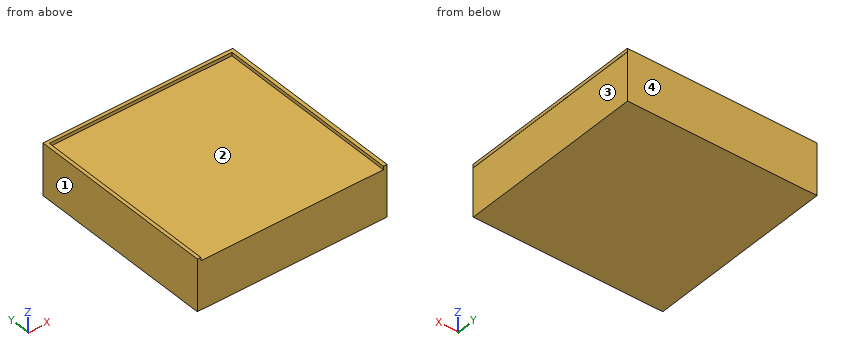
```python
from build123d import *

# Parameters (mm, degrees)
F2_DEPTH = 1
F0_W     = 55
F0_H     = 55
F3_DEPTH = 14


with BuildPart() as f2:
    # F1 (on face) → F2 (new body)
    with BuildSketch(Plane.XY):
        Polygon((1, -1), (54, -1), (54, -55), (55.060755, -55), (55.060755, 0), (0, 0), (0, -55), (1, -55), align=None)
    extrude(amount=F2_DEPTH)

    # F0 (on Top) → F3 (join)
    with BuildSketch(Plane.XY):
        with Locations((27.5, -27.5)):
            Rectangle(F0_W, F0_H)
    extrude(amount=-F3_DEPTH)


solid = f2.part
```
Geometry check sheet. Reference: the model listing, model coordinates, mm. Face numbers are marked on the shaded views. Coordinates: 2 decimals unless noted, no trailing zeros. Write each loop counter-clockwise with the first axis right and the second up, starting at its lowest first coordinate (ties: lowest second). Pieces come first, ordered by that corner, then holes. Notation, with made-up numbers: (81.5, 71) -> (99.5, 71) arc R34 ccw to (99.5, 108) -> close; hole circle Ø6 at (82.25, 30). An arc over 180 degrees is marked (long way). Use CSV: the item, a comma, the result in double quotes. Start each with the question number.
Item 1: Cross-section at B-B, the plane x = 12. Record the cut outline in (y, z).
Item 2: Thickness scan on line 1 (X direction, y = -35.5, z = -10.25); line 2 (Z direction, x = 2, y = -22). Record the ranges inside material, lowest first.
Item 3: Depth check by flat-ended pin: pin 1 Ø16 at (x, y) = (28.5, -38.5) entering from +Z; pin 2 Ø7 at (y, z) = (-23.5, -5.5) entering from +X. Enter the tip coordinate at first touch or a pass-through.
Item 4: Mould release check, pull along X, two halves, no side actions. Record for the marked faces 1, 2, 3 and 4: released by +X, released by -X, zero draft, split by the parting line, or undercut.
Item 5: Cross-section at A-A, the plane y = -36. Record the cut outline in (x, z).
Answers:
1,outline,"(-55, -14) -> (0, -14) -> (0, 1) -> (-1, 1) -> (-1, 0) -> (-55, 0) -> close"
2,line 1,"0 to 55"
2,line 2,"-14 to 0"
3,pin 1,"z = 0"
3,pin 2,"x = 55"
4,face 1,"released by -X"
4,face 2,"undercut"
4,face 3,"released by +X"
4,face 4,"zero draft"
5,outline,"(0, -14) -> (55, -14) -> (55, 0) -> (55.06, 0) -> (55.06, 1) -> (54, 1) -> (54, 0) -> (1, 0) -> (1, 1) -> (0, 1) -> close"
